Geometry check sheet. Reference: the model listing, model coordinates, mm. A direction names the side the tool comes from. Round coordinates to 2 decimals unless told otherwise and drop trailing zeros. Use one line per item in the form item = value. Start each with the question number.
1. Go/stop test with flat-tipped pins: pin 1 (5 mm diameter, centred on x = 20, y = 83, fed in from +Z); pin 2 (7 mm diameter, centred on y = 0, z = 12.7, fed in from -X). Record where each tip stops, or that it passes through.
2. Set-up check for faces 3 (the cylindrical face through (86.245, 83.795, 11.824)), 4 (the flat face through (-16, -80, 15.088)), 5 (the cylindrical face through (-97.528, -69.205, 11.951)): record each of +Z, -Z, +X, -X, +Y, -Y from which the full face is reachable in a straight line by a thin tool's end or side.
3. Draft check along Y on faces 1 (the conical face through (-0.3, 85.408, 13.653)), 2 (the cylindrical face through (-91.555, 83.795, 11.824)). Enter one of: pulls with the +Y half, pulls with the -Y half, needs draft (parallel to the pull), parting line crosses it, or undercut.
4. Material ranges on line 1 (Z direction, x = 63, y = 97); line 2 (X direction, y = 92, z = 12.7); line 3 (Y direction, x = 86, z = 6.25), recorded low to high.
```python
from build123d import *

# Parameters (mm, degrees)
SKETCH1_W                                        = 215.9
SKETCH1_H                                        = 215.9
BOSS_EXTRUDE1_DEPTH                              = 25.4
F_1_2_20_TAPPED_HOLE1_D                          = 11.50874
F_1_2_20_TAPPED_HOLE1_CSINK_D                    = 13.97
F_1_2_20_TAPPED_HOLE1_CSINK_ANGLE                = 82
CBORE_FOR_3_8_SOCKET_HEAD_CAP_SCREW1_D           = 10.3124
CBORE_FOR_3_8_SOCKET_HEAD_CAP_SCREW1_CBORE_D     = 15.875
CBORE_FOR_3_8_SOCKET_HEAD_CAP_SCREW1_CBORE_DEPTH = 10.3124
F_1_2_20_TAPPED_HOLE2_AT_2_COUNT                 = 2
F_1_2_20_TAPPED_HOLE2_AT_2_PITCH                 = 63.5
F_1_2_20_TAPPED_HOLE2_AT_3_COUNT                 = 2
F_1_2_20_TAPPED_HOLE2_AT_3_PITCH                 = 63.5
CIRPATTERN1_COUNT                                = 2
CIRPATTERN1_ANGLE                                = 90


with BuildPart() as part:
    # Sketch1 → Boss-Extrude1 (new body)
    with BuildSketch(Plane.XY):
        Rectangle(SKETCH1_W, SKETCH1_H)
    extrude(amount=BOSS_EXTRUDE1_DEPTH)

    # 1/2-20 Tapped Hole1 (through all)
    with Locations(Plane.XY.offset(25.4)):
        with Locations((-88.9, -88.9), (88.9, 88.9), (-88.9, 88.9), (88.9, -88.9)):
            CounterSinkHole(F_1_2_20_TAPPED_HOLE1_D / 2, F_1_2_20_TAPPED_HOLE1_CSINK_D / 2, counter_sink_angle=F_1_2_20_TAPPED_HOLE1_CSINK_ANGLE)

    # CBORE for 3/8 Socket Head Cap Screw1 (through all)
    with Locations(Plane.XY.offset(25.4)):
        with Locations((-58.371664787, 58.371664787), (-79.73717696, -21.365512173), (-21.365512173, -79.73717696), (58.371664787, -58.371664787), (79.73717696, 21.365512173), (21.365512173, 79.73717696)):
            CounterBoreHole(CBORE_FOR_3_8_SOCKET_HEAD_CAP_SCREW1_D / 2, CBORE_FOR_3_8_SOCKET_HEAD_CAP_SCREW1_CBORE_D / 2, CBORE_FOR_3_8_SOCKET_HEAD_CAP_SCREW1_CBORE_DEPTH)

    # Sketch6 → 1/2-20 Tapped Hole2 (revolve, cut)
    with BuildSketch(Plane(origin=(-107.95, 0, 12.7), x_dir=(0, 0, 1), z_dir=(0, 1, 0))):
        Polygon((0, 0), (0, 23.14257432), (5.75437, 19.685), (5.75437, 1.415677873), (6.985, 0), align=None)
    f_1_2_20_tapped_hole2 = revolve(axis=Axis((-114.3, 0, 12.7), (1, 0, 0)), mode=Mode.SUBTRACT)

    # 1/2-20 Tapped Hole2 at 2: 1/2-20 Tapped Hole2 ×2
    with Locations(*[(0, i * F_1_2_20_TAPPED_HOLE2_AT_2_PITCH, 0) for i in range(1, F_1_2_20_TAPPED_HOLE2_AT_2_COUNT)]):
        add(f_1_2_20_tapped_hole2, mode=Mode.SUBTRACT)

    # 1/2-20 Tapped Hole2 at 3: 1/2-20 Tapped Hole2 ×2
    with Locations(*[(0, -i * F_1_2_20_TAPPED_HOLE2_AT_3_PITCH, 0) for i in range(1, F_1_2_20_TAPPED_HOLE2_AT_3_COUNT)]):
        add(f_1_2_20_tapped_hole2, mode=Mode.SUBTRACT)

    # CirPattern1: 1/2-20 Tapped Hole2 ×2 about axis
    cirpattern1_axis = Axis((0, 0, -1.27), (0, 0, -1))
    for i in range(1, CIRPATTERN1_COUNT):
        add(f_1_2_20_tapped_hole2.rotate(cirpattern1_axis, i * CIRPATTERN1_ANGLE / (CIRPATTERN1_COUNT - 1)), mode=Mode.SUBTRACT)

    # CirPattern1 copy 1 sketch → CirPattern1 copy 1 (revolve, cut)
    with BuildSketch(Plane(origin=(63.5, 107.95, 12.7), x_dir=(0, 0, 1), z_dir=(1, 0, 0))):
        Polygon((0, 0), (0, 23.14257432), (5.75437, 19.685), (5.75437, 1.415677873), (6.985, 0), align=None)
    revolve(axis=Axis((63.5, 114.3, 12.7), (0, -1, 0)), mode=Mode.SUBTRACT)

    # CirPattern1 copy 2 sketch → CirPattern1 copy 2 (revolve, cut)
    with BuildSketch(Plane(origin=(-63.5, 107.95, 12.7), x_dir=(0, 0, 1), z_dir=(1, 0, 0))):
        Polygon((0, 0), (0, 23.14257432), (5.75437, 19.685), (5.75437, 1.415677873), (6.985, 0), align=None)
    revolve(axis=Axis((-63.5, 114.3, 12.7), (0, -1, 0)), mode=Mode.SUBTRACT)


solid = part.part
```
Reported:
q1.pin_1 = 15.09
q1.pin_2 = -86.91
q2.face_3 = +Z, -Z
q2.face_4 = +Z
q2.face_5 = -X
q3.face_1 = pulls with the +Y half
q3.face_2 = undercut
q4.line_1 = 0 to 6.97, 18.43 to 25.4
q4.line_2 = -107.95 to -93.75, -84.05 to -69.25, -57.75 to -5.75, 5.75 to 57.75, 69.25 to 84.05, 93.75 to 107.95
q4.line_3 = -107.95 to -93.87, -83.93 to 83.93, 93.87 to 107.95
